The model under review builds one solid part; all positions refer to its coordinate system, in mm. A direction names the side the tool comes from. Round coordinates to 2 decimals unless told otherwise and drop trailing zeros. Write each loop counter-clockwise with the first axis right and the second up, starting at its lowest first coordinate (ties: lowest second). Pieces come first, ordered by that corner, then holes. Notation, with made-up numbers: (40.5, -9.75) -> (72.5, -9.75) arc R24 ccw to (72.5, 15.25) -> close; hole circle Ø9 at (21.25, -15.5). An arc over 180 degrees is marked (long way). Answer as a JSON object with one key per item and string values. Group by question number.
1) We need section A-A, the plane y = 0. Count the separate pieces of the cut face and the enclosed holes in it, then the cut area to 3 significant figures.
2) We need section B-B, the plane x = 45. Write out the cut boundary in (y, z) (3 decimals).
3) We need section C-C, the plane x = 15. Write out the cut boundary in (y, z).
4) To check wall thickness, follow probe 1 along Y at (x, z) = (-45, 1.6); probe 2 along Y at (x, z) = (-45, 7.9) (3 decimals); probe 3 along Z at (x, y) = (18.5, 9). State the ranges of each line that lie inside material, in increasing order. Write a range as [from, to].
5) Machinability: for faces 4 (the cylindrical face through (-44.82, 11.93, 9.4)), 5 (the flat face through (5, 0, 14)), 6 (the flat face through (-42, -5, 10)), which of the approach directions +Z, -Z, +X, -X, +Y, -Y give a long, thin tool a straight path to every point of the face, cutting with its end or side? Answer none if there is none.
6) Insertion check: pin 1 Ø4 at (x, y) = (-37, 9.5) entering from -Z; pin 2 Ø8 at (y, z) = (3.5, 17.5) entering from -X; pin 3 Ø2.5 at (x, y) = (-2.5, -15) entering from -Z; pin 4 Ø2 at (x, y) = (-30.5, -4) entering from +Z. Each pin has a flat end and moves straight along its axis. Give the tip position at first contact, or say it passes through.
7) Mouldability with a two-part tool opening along X and no side actions: class faces 1 (the cylindrical face through (44.82, -11.93, 9.4)), 2 (the flat face through (-7.846, -0.28, 5.07)), 3 (the cylindrical face through (29.4, 16.45, 29.43)) as pulls with the +X half, pulls with the -X half, needs draft (parallel to the pull), parting line crosses it, or undercut.
from build123d import *

# Parameters (mm, degrees)
F0_W           = 60
F0_H           = 40
F1_DEPTH       = 30
F3_DEPTH       = 40.001
F4_R           = 15
F5_DEPTH       = 40
F6_W           = 25
F6_H           = 10
F7_DEPTH       = 30
F9_D           = 5.5
F9_CBORE_D     = 9.75
F9_CBORE_DEPTH = 5
F10_T1_DEPTH   = 13
F10_T3_DEPTH   = 28
F10_T5_DEPTH   = 21
F10_T7_DEPTH   = 33
F10_T9_DEPTH   = 8
F10_T11_DEPTH  = 56
F10_T13_DEPTH  = 8
F10_S17_W      = 2
F10_S17_H      = 2
F10_T18_DEPTH  = 2
F10_S23_W      = 2
F10_S23_H      = 2
F10_T24_DEPTH  = 2
F10_S29_W      = 2
F10_S29_H      = 2
F10_T30_DEPTH  = 2
F10_S35_W      = 2
F10_S35_H      = 2
F10_T36_DEPTH  = 2
F10_S41_W      = 2
F10_S41_H      = 2
F10_T42_DEPTH  = 2
F10_S47_W      = 2
F10_S47_H      = 2
F10_T48_DEPTH  = 2
F10_T51_DEPTH  = 8
F10_T53_DEPTH  = 21
F10_T56_ANGLE  = 90
F10_T58_ANGLE  = 90


# Not quite as in the source:
# - a fillet or chamfer that OpenCascade refuses, or shapes differently, is made with other operations: its cross-section is extruded or revolved along the edge and cut away or added


with BuildPart() as f1:
    # F0 (on Top) → F1 (new body)
    with BuildSketch(Plane.XY):
        Rectangle(F0_W, F0_H)
    extrude(amount=F1_DEPTH)

    # F2 (on face) → F3 (cut, through all)
    with BuildSketch(Plane.XZ.offset(20)):
        Polygon((-5, 10), (-10.7735026919, 0), (10.7735026919, 0), (5, 10), (5, 20), (-5, 20), align=None)
    extrude(amount=-F3_DEPTH, mode=Mode.SUBTRACT)

    # F4 (on Right) → F5 (cut, symmetric)
    with BuildSketch(Plane.YZ):
        with Locations((0, 30)):
            Circle(F4_R)
    extrude(amount=F5_DEPTH, both=True, mode=Mode.SUBTRACT)

    # F6 (on face) → F7 (join)
    with BuildSketch(Plane.YZ.offset(30)):
        with Locations((0, 5)):
            Rectangle(F6_W, F6_H)
    extrude(amount=F7_DEPTH)

    # F9 (through all)
    with Locations(Plane.XY.offset(10)):
        with Locations((45, 0)):
            CounterBoreHole(F9_D / 2, F9_CBORE_D / 2, F9_CBORE_DEPTH)

    # F10: fillet of radius 2 on 18 edges, made by hand

    # F10_s2 → F10_t1 (cut)
    with BuildSketch(Plane.XY.offset(-5)):
        with BuildLine():
            ThreePointArc((58, -12.5), (59.4142135624, -11.9142135624), (60, -10.5))
            Line((60, -10.5), (60, -12.5))
            Line((60, -12.5), (58, -12.5))
        make_face()
        with BuildLine():
            ThreePointArc((60, 10.5), (59.4142135624, 11.9142135624), (58, 12.5))
            Line((58, 12.5), (60, 12.5))
            Line((60, 12.5), (60, 10.5))
        make_face()
    extrude(amount=F10_T1_DEPTH, mode=Mode.SUBTRACT)

    # F10_s4 → F10_t3 (cut)
    with BuildSketch(Plane.YZ.offset(30)):
        with BuildLine():
            ThreePointArc((-12.5, 8), (-11.9142135624, 9.4142135624), (-10.5, 10))
            Line((-10.5, 10), (-12.5, 10))
            Line((-12.5, 10), (-12.5, 8))
        make_face()
        with BuildLine():
            ThreePointArc((12.5, 8), (11.9142135624, 9.4142135624), (10.5, 10))
            Line((10.5, 10), (12.5, 10))
            Line((12.5, 10), (12.5, 8))
        make_face()
    extrude(amount=F10_T3_DEPTH, mode=Mode.SUBTRACT)

    # F10_s6 → F10_t5 (cut)
    with BuildSketch(Plane.XZ.offset(-10.5)):
        with BuildLine():
            ThreePointArc((60, 8), (59.4142135624, 9.4142135624), (58, 10))
            Line((58, 10), (60, 10))
            Line((60, 10), (60, 8))
        make_face()
    extrude(amount=F10_T5_DEPTH, mode=Mode.SUBTRACT)

    # F10_s8 → F10_t7 (cut)
    with BuildSketch(Plane.XY.offset(-5)):
        with BuildLine():
            ThreePointArc((30, -18), (29.4142135624, -19.4142135624), (28, -20))
            Line((28, -20), (30, -20))
            Line((30, -20), (30, -18))
        make_face()
        with BuildLine():
            ThreePointArc((28, 20), (29.4142135624, 19.4142135624), (30, 18))
            Line((30, 18), (30, 20))
            Line((30, 20), (28, 20))
        make_face()
        with BuildLine():
            ThreePointArc((-30, -18), (-29.4142135624, -19.4142135624), (-28, -20))
            Line((-28, -20), (-30, -20))
            Line((-30, -20), (-30, -18))
        make_face()
        with BuildLine():
            ThreePointArc((-28, 20), (-29.4142135624, 19.4142135624), (-30, 18))
            Line((-30, 18), (-30, 20))
            Line((-30, 20), (-28, 20))
        make_face()
    extrude(amount=F10_T7_DEPTH, mode=Mode.SUBTRACT)

    # F10_s10 → F10_t9 (cut)
    with BuildSketch(Plane.XZ.offset(10)):
        with BuildLine():
            ThreePointArc((30, 28), (29.4142135624, 29.4142135624), (28, 30))
            Line((28, 30), (30, 30))
            Line((30, 30), (30, 28))
        make_face()
        with BuildLine():
            ThreePointArc((-30, 28), (-29.4142135624, 29.4142135624), (-28, 30))
            Line((-28, 30), (-30, 30))
            Line((-30, 30), (-30, 28))
        make_face()
    extrude(amount=F10_T9_DEPTH, mode=Mode.SUBTRACT)

    # F10_s12 → F10_t11 (cut)
    with BuildSketch(Plane.YZ.offset(-28)):
        with BuildLine():
            ThreePointArc((20, 28), (19.4142135624, 29.4142135624), (18, 30))
            Line((18, 30), (20, 30))
            Line((20, 30), (20, 28))
        make_face()
        with BuildLine():
            ThreePointArc((-20, 28), (-19.4142135624, 29.4142135624), (-18, 30))
            Line((-18, 30), (-20, 30))
            Line((-20, 30), (-20, 28))
        make_face()
    extrude(amount=F10_T11_DEPTH, mode=Mode.SUBTRACT)

    # F10_s14 → F10_t13 (cut)
    with BuildSketch(Plane.XZ.offset(-18)):
        with BuildLine():
            ThreePointArc((-30, 28), (-29.4142135624, 29.4142135624), (-28, 30))
            Line((-28, 30), (-30, 30))
            Line((-30, 30), (-30, 28))
        make_face()
        with BuildLine():
            ThreePointArc((28, 30), (29.4142135624, 29.4142135624), (30, 28))
            Line((30, 28), (30, 30))
            Line((30, 30), (28, 30))
        make_face()
    extrude(amount=F10_T13_DEPTH, mode=Mode.SUBTRACT)


with BuildPart() as f10_tool16:
    # F10_s17 → F10_t18 (new body)
    with BuildSketch(Plane.XY.offset(8)):
        with Locations((59, -11.5)):
            Rectangle(F10_S17_W, F10_S17_H)
    extrude(amount=F10_T18_DEPTH)

    # F10_s19 → F10_t20 (revolve, cut)
    with BuildSketch(Plane(origin=(58, -10.5, 8), x_dir=(-0.7071067812, 0.7071067812, 0), z_dir=(0.7071067812, 0.7071067812, 0))):
        with BuildLine():
            ThreePointArc((0, -2), (2, 0), (0, 2))
            Line((0, 2), (0, -2))
        make_face()
    revolve(axis=Axis((58, -10.5, 8), (0, 0, 1)), mode=Mode.SUBTRACT)


with BuildPart() as f1_1:
    add(f1.part)

    # F10_t15: cut F10_tool16
    add(f10_tool16.part, mode=Mode.SUBTRACT)


with BuildPart() as f10_tool22:
    # F10_s23 → F10_t24 (new body)
    with BuildSketch(Plane.XY.offset(8)):
        with Locations((59, 11.5)):
            Rectangle(F10_S23_W, F10_S23_H)
    extrude(amount=F10_T24_DEPTH)

    # F10_s25 → F10_t26 (revolve, cut)
    with BuildSketch(Plane(origin=(58, 10.5, 8), x_dir=(-0.7071067812, -0.7071067812, 0), z_dir=(-0.7071067812, 0.7071067812, 0))):
        with BuildLine():
            ThreePointArc((0, -2), (2, 0), (0, 2))
            Line((0, 2), (0, -2))
        make_face()
    revolve(axis=Axis((58, 10.5, 8), (0, 0, 1)), mode=Mode.SUBTRACT)


with BuildPart() as f1_2:
    add(f1_1.part)

    # F10_t21: cut F10_tool22
    add(f10_tool22.part, mode=Mode.SUBTRACT)


with BuildPart() as f10_tool28:
    # F10_s29 → F10_t30 (new body)
    with BuildSketch(Plane.XY.offset(28)):
        with Locations((29, -19)):
            Rectangle(F10_S29_W, F10_S29_H)
    extrude(amount=F10_T30_DEPTH)

    # F10_s31 → F10_t32 (revolve, cut)
    with BuildSketch(Plane(origin=(28, -18, 28), x_dir=(-0.7071067812, 0.7071067812, 0), z_dir=(0.7071067812, 0.7071067812, 0))):
        with BuildLine():
            ThreePointArc((0, -2), (2, 0), (0, 2))
            Line((0, 2), (0, -2))
        make_face()
    revolve(axis=Axis((28, -18, 28), (0, 0, 1)), mode=Mode.SUBTRACT)


with BuildPart() as f1_3:
    add(f1_2.part)

    # F10_t27: cut F10_tool28
    add(f10_tool28.part, mode=Mode.SUBTRACT)


with BuildPart() as f10_tool34:
    # F10_s35 → F10_t36 (new body)
    with BuildSketch(Plane.YZ.offset(-28)):
        with Locations((-19, 29)):
            Rectangle(F10_S35_W, F10_S35_H)
    extrude(amount=-F10_T36_DEPTH)

    # F10_s37 → F10_t38 (revolve, cut)
    with BuildSketch(Plane(origin=(-28, -18, 28), x_dir=(0, 0.7071067812, -0.7071067812), z_dir=(0, 0.7071067812, 0.7071067812))):
        with BuildLine():
            ThreePointArc((0, -2), (2, 0), (0, 2))
            Line((0, 2), (0, -2))
        make_face()
    revolve(axis=Axis((-28, -18, 28), (-1, 0, 0)), mode=Mode.SUBTRACT)


with BuildPart() as f1_4:
    add(f1_3.part)

    # F10_t33: cut F10_tool34
    add(f10_tool34.part, mode=Mode.SUBTRACT)


with BuildPart() as f10_tool40:
    # F10_s41 → F10_t42 (new body)
    with BuildSketch(Plane.XZ.offset(-18)):
        with Locations((29, 29)):
            Rectangle(F10_S41_W, F10_S41_H)
    extrude(amount=-F10_T42_DEPTH)

    # F10_s43 → F10_t44 (revolve, cut)
    with BuildSketch(Plane(origin=(28, 18, 28), x_dir=(-0.7071067812, 0, -0.7071067812), z_dir=(0.7071067812, 0, -0.7071067812))):
        with BuildLine():
            ThreePointArc((0, -2), (2, 0), (0, 2))
            Line((0, 2), (0, -2))
        make_face()
    revolve(axis=Axis((28, 18, 28), (0, 1, 0)), mode=Mode.SUBTRACT)


with BuildPart() as f1_5:
    add(f1_4.part)

    # F10_t39: cut F10_tool40
    add(f10_tool40.part, mode=Mode.SUBTRACT)


with BuildPart() as f10_tool46:
    # F10_s47 → F10_t48 (new body)
    with BuildSketch(Plane.XZ.offset(-18)):
        with Locations((-29, 29)):
            Rectangle(F10_S47_W, F10_S47_H)
    extrude(amount=-F10_T48_DEPTH)

    # F10_s49 → F10_t50 (revolve, cut)
    with BuildSketch(Plane(origin=(-28, 18, 28), x_dir=(0.7071067812, 0, -0.7071067812), z_dir=(0.7071067812, 0, 0.7071067812))):
        with BuildLine():
            ThreePointArc((0, -2), (2, 0), (0, 2))
            Line((0, 2), (0, -2))
        make_face()
    revolve(axis=Axis((-28, 18, 28), (0, 1, 0)), mode=Mode.SUBTRACT)


with BuildPart() as f1_6:
    add(f1_5.part)

    # F10_t45: cut F10_tool46
    add(f10_tool46.part, mode=Mode.SUBTRACT)

    # F10_s52 → F10_t51 (join)
    with BuildSketch(Plane.XY):
        with BuildLine():
            ThreePointArc((30, -14.5), (30.5857864376, -13.0857864376), (32, -12.5))
            Line((32, -12.5), (30, -12.5))
            Line((30, -12.5), (30, -14.5))
        make_face()
        with BuildLine():
            ThreePointArc((30, 14.5), (30.5857864376, 13.0857864376), (32, 12.5))
            Line((32, 12.5), (30, 12.5))
            Line((30, 12.5), (30, 14.5))
        make_face()
    extrude(amount=F10_T51_DEPTH)

    # F10_s54 → F10_t53 (join)
    with BuildSketch(Plane.XZ.offset(-10.5)):
        with BuildLine():
            ThreePointArc((30, 12), (30.5857864376, 10.5857864376), (32, 10))
            Line((32, 10), (30, 10))
            Line((30, 10), (30, 12))
        make_face()
    extrude(amount=F10_T53_DEPTH)

    # F10_s55 → F10_t56 (revolve)
    with BuildSketch(Plane.XY.offset(8)):
        with BuildLine():
            ThreePointArc((30, 14.5), (30.5857864376, 13.0857864376), (32, 12.5))
            Line((32, 12.5), (30, 12.5))
            Line((30, 12.5), (30, 14.5))
        make_face()
    revolve(axis=Axis((30, 10.5, 8), (1, 0, 0)), revolution_arc=F10_T56_ANGLE)

    # F10_s57 → F10_t58 (revolve)
    with BuildSketch(Plane.XY.offset(8)):
        with BuildLine():
            ThreePointArc((30, -14.5), (30.5857864376, -13.0857864376), (32, -12.5))
            Line((32, -12.5), (30, -12.5))
            Line((30, -12.5), (30, -14.5))
        make_face()
    revolve(axis=Axis((30, -10.5, 8), (-1, 0, 0)), revolution_arc=F10_T58_ANGLE)

    # F11: F1 across plane


with BuildPart() as f1_7:
    add(f1_6.part)
    add(f1_6.part.mirror(Plane.YZ))


solid = f1_7.part
Here are the results:
{
 "1": {"separate pieces": "4", "enclosed holes": "0", "area": "1,140 mm^2"},
 "2": {"outline": "(-12.5, 0) -> (-2.75, 0) -> (-2.75, 5) -> (-4.875, 5) -> (-4.875, 10) -> (-10.5, 10) arc R2 ccw to (-12.5, 8) -> close; (2.75, 0) -> (12.5, 0) -> (12.5, 8) arc R2 ccw to (10.5, 10) -> (4.875, 10) -> (4.875, 5) -> (2.75, 5) -> close"},
 "3": {"outline": "(-20, 0) -> (20, 0) -> (20, 28) arc R2 ccw to (18, 30) -> (15, 30) arc R15 cw to (-15, 30) -> (-18, 30) arc R2 ccw to (-20, 28) -> close"},
 "4": {"probe 1": "y = [-12.5, -2.75], [2.75, 12.5]", "probe 2": "y = [-12.5, -4.875], [4.875, 12.5]", "probe 3": "z = [0, 18]"},
 "5": {"face 4": "+Z, -X, +Y", "face 5": "-Z, +Y, -Y", "face 6": "+Z, -X, +Y, -Y"},
 "6": {"pin 1": "stops at z = 0", "pin 2": "stops at x = -30", "pin 3": "stops at z = 20", "pin 4": "stops at z = 15.81"},
 "7": {"face 1": "needs draft", "face 2": "undercut", "face 3": "pulls with the +X half"}
}
